Could you check a few things on this model? Use its own coordinates, in mm. Give positions to 0.01 mm unless a question says otherwise; leave off trailing zeros. Write each loop counter-clockwise with the first axis right and the second up, starting at its lowest first coordinate (ties: lowest second). Pieces come first, ordered by that corner, then holes. Notation, with made-up numbers: M 77,29.5 L 100,29.5 A26 cw 100,57.5 Z; hole C -19,57.5 d9. An arc over 180 degrees is marked long. Use one line per item in the form item = value.
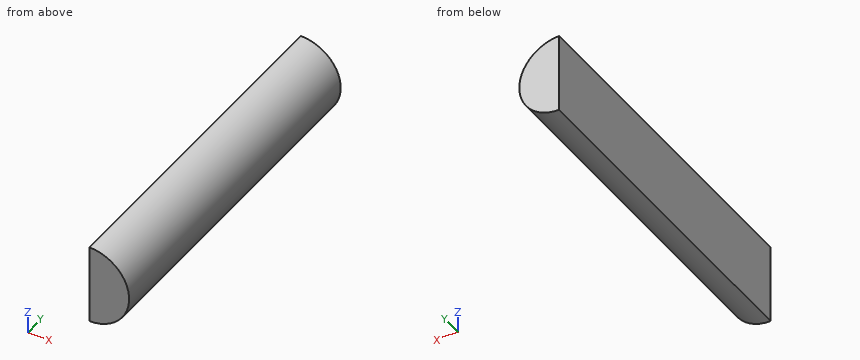
from build123d import *

# Parameters (mm, degrees)
SKETCH1_R           = 2.38125
BOSS_EXTRUDE1_DEPTH = 1.5875
SKETCH2_R           = 3.175
BOSS_EXTRUDE2_DEPTH = 1.5875
SKETCH3_R           = 2.38125
BOSS_EXTRUDE3_DEPTH = 19.05
SKETCH4_R           = 3.175
BOSS_EXTRUDE4_DEPTH = 1.5875
SKETCH5_R           = 2.38125
BOSS_EXTRUDE5_DEPTH = 1.5875
SKETCH9_W           = 27.857962544
SKETCH9_H           = 18.98631043
SKETCH9_R           = 2.38125
CUT_EXTRUDE4_DEPTH  = 28.662025878
SKETCH12_W          = 2.976246955
SKETCH12_H          = 4.951375607
CUT_EXTRUDE5_DEPTH  = 23.746254865


with BuildPart() as part:
    # Sketch1 → Boss-Extrude1 (new body)
    with BuildSketch(Plane(origin=(0, 0, 0), x_dir=(1, 0, 0), z_dir=(0, 1, 0))):
        with BuildLine():
            Line((9.398005644, 4.762076723), (-6.35, 4.7625))
            ThreePointArc((-6.35, 4.7625), (-11.020584629, 0.931152767), (-8.176363381, -4.398386414))
            ThreePointArc((-8.176363381, -4.398386414), (-5.292234705, -6.221263486), (-3.181508348, -8.901918869))
            ThreePointArc((-3.181508348, -8.901918869), (1.849687492, -11.693035316), (6.504625866, -8.311495529))
            ThreePointArc((6.504625866, -8.311495529), (8.146827792, -5.96033805), (10.67447942, -4.60544104))
            ThreePointArc((10.67447942, -4.60544104), (14.180390361, 0.643024113), (9.398005644, 4.762076723))
        make_face()
        with Locations(Location((-6.35, 0, 0), (0, 0, 270))):
            Circle(SKETCH1_R, mode=Mode.SUBTRACT)
        with Locations(Location((9.4615, 0, 0), (0, 0, 270))):
            Circle(SKETCH1_R, mode=Mode.SUBTRACT)
        with Locations(Location((1.524, -6.35, 0), (0, 0, 270))):
            Circle(SKETCH1_R, mode=Mode.SUBTRACT)
    extrude(amount=BOSS_EXTRUDE1_DEPTH)

    # Sketch2 → Boss-Extrude2 (add)
    with BuildSketch(Plane.XZ):
        with Locations(Location((1.524, 6.35, 0), (0, 0, 90))):
            Circle(SKETCH2_R)
    extrude(amount=BOSS_EXTRUDE2_DEPTH)

    # Sketch3 → Boss-Extrude3 (add)
    with BuildSketch(Plane(origin=(0, 0, 0), x_dir=(1, 0, 0), z_dir=(0, 1, 0))):
        with Locations(Location((1.524, -6.35, 0), (0, 0, 90))):
            Circle(SKETCH3_R)
    extrude(amount=BOSS_EXTRUDE3_DEPTH)

    # Sketch4 → Boss-Extrude4 (add)
    with BuildSketch(Plane(origin=(0, 19.05, 0), x_dir=(1, 0, 0), z_dir=(0, 1, 0))):
        with Locations(Location((1.524, -6.35, 0), (0, 0, 270))):
            Circle(SKETCH4_R)
    extrude(amount=-BOSS_EXTRUDE4_DEPTH)


with BuildPart() as body_2:
    # Sketch5 → Boss-Extrude5 (new body)
    with BuildSketch(Plane.XZ.offset(-17.4625)):
        with BuildLine():
            ThreePointArc((-8.176363381, 4.398386414), (-11.020584629, -0.931152767), (-6.35, -4.7625))
            Line((-6.35, -4.7625), (9.4615, -4.7625))
            ThreePointArc((9.4615, -4.7625), (14.184572051, -0.611552653), (10.67447942, 4.60544104))
            ThreePointArc((10.67447942, 4.60544104), (8.146827792, 5.96033805), (6.504625866, 8.311495529))
            ThreePointArc((6.504625866, 8.311495529), (1.849687492, 11.693035316), (-3.181508348, 8.901918869))
            ThreePointArc((-3.181508348, 8.901918869), (-5.292234705, 6.221263486), (-8.176363381, 4.398386414))
        make_face()
        with Locations(Location((-6.35, 0, 0), (0, 0, 90))):
            Circle(SKETCH5_R, mode=Mode.SUBTRACT)
        with Locations(Location((9.4615, 0, 0), (0, 0, 90))):
            Circle(SKETCH5_R, mode=Mode.SUBTRACT)
        with Locations(Location((1.524, 6.35, 0), (0, 0, 270))):
            Circle(SKETCH5_R, mode=Mode.SUBTRACT)
    extrude(amount=BOSS_EXTRUDE5_DEPTH)


with BuildPart() as cut_extrude4_tool:
    # Sketch9 → Cut-Extrude4 (new, through all)
    with BuildSketch(Plane.XZ.offset(1.5875)):
        with Locations((1.177973605, 3.738325546)):
            Rectangle(SKETCH9_W, SKETCH9_H)
        with Locations(Location((1.524, 6.35, 0), (0, 0, 270))):
            Circle(SKETCH9_R, mode=Mode.SUBTRACT)
    extrude(amount=-CUT_EXTRUDE4_DEPTH)


with BuildPart() as part_1:
    add(part.part)

    # Cut-Extrude4: cut by cut_extrude4_tool
    add(cut_extrude4_tool.part, mode=Mode.SUBTRACT)

    # Sketch12 → Cut-Extrude5 (cut, through all)
    with BuildSketch(Plane.XZ.offset(1.5875)):
        with Locations((0.035876522, 6.255562197)):
            Rectangle(SKETCH12_W, SKETCH12_H)
    extrude(amount=-CUT_EXTRUDE5_DEPTH, mode=Mode.SUBTRACT)


with BuildPart() as body_2_1:
    add(body_2.part)

    # Cut-Extrude4: cut by cut_extrude4_tool
    add(cut_extrude4_tool.part, mode=Mode.SUBTRACT)


solid = part_1.part
1) I want a section at B-B, the plane x = 2.05. Please give me the cut outline in (y, z).
Checked values:
outline = M -1.59,4.03 L 19.05,4.03 L 19.05,8.67 L -1.59,8.67 Z
2) I want a section at C-C, the plane z = 5.1. Please give me the cut outline in (x, y).
Checked values:
outline = M 1.52,-1.59 L 3.55,-1.59 L 3.55,19.05 L 1.52,19.05 Z
3) I want a section at A-A, the plane y = 1. Please give me the cut outline in (x, z).
Checked values:
outline = M 1.52,3.97 A2.38 ccw 1.52,8.73 Z
4) If I drill on L1, parallel to X at y = 9, z = 6.45; L2, parallel to Z at x = 2.1, y = 2.5; L3, parallel to Z at x = 3.4, y = 2.5, over which ranges is the centre line in solid material (lowest first)?
Checked values:
L1 = 1.52 to 3.9
L2 = 4.04 to 8.66
L3 = 4.88 to 7.82
